Here's how the part is built. I have some questions about the finished solid (model axes, mm). Face numbers are marked on the shaded views. A direction names the side the tool comes from. Coordinates: 2 decimals unless noted, no trailing zeros. Write each loop counter-clockwise with the first axis right and the second up, starting at its lowest first coordinate (ties: lowest second). Pieces come first, ordered by that corner, then holes. Notation, with made-up numbers: M 14.5,-11 L 28.5,-11 A12 ccw 28.5,12 Z; hole C 19.5,33.25 d7. An arc over 180 degrees is marked long. Use a Markdown table: item, result.
```python
from build123d import *

# Parameters (mm, degrees)
CROQUIS1_W              = 111.196890842
CROQUIS1_H              = 104.63014532
SALIENTE_EXTRUIR1_DEPTH = 25
SALIENTE_EXTRUIR2_DEPTH = 25
MATRIZL4_COUNT          = 2
MATRIZL4_PITCH          = 50
MATRIZL5_COUNT          = 2
MATRIZL5_PITCH          = 50
CROQUIS3_R              = 50.793115706
CORTAR_EXTRUIR4_DEPTH   = 120


with BuildPart() as part:
    # Croquis1 → Saliente-Extruir1 (new body)
    with BuildSketch(Plane.XY):
        Rectangle(CROQUIS1_W, CROQUIS1_H)
    saliente_extruir1 = extrude(amount=SALIENTE_EXTRUIR1_DEPTH)

    # Croquis2 → Saliente-Extruir2 (add)
    with BuildSketch(Plane.XY.offset(25)):
        Polygon((-3.132824134, -80.10377536), (81.011557784, -3.059075666), (4.937773514, 80.024920806), (-79.206608404, 2.980221112), align=None)
    saliente_extruir2 = extrude(amount=SALIENTE_EXTRUIR2_DEPTH)

    # MatrizL4: Saliente-Extruir1, Saliente-Extruir2 ×2
    with Locations(*[(0, 0, i * MATRIZL4_PITCH) for i in range(1, MATRIZL4_COUNT)]):
        add(saliente_extruir1)
        add(saliente_extruir2)

    # MatrizL5: Saliente-Extruir2 ×2
    with Locations(*[(0, 0, -i * MATRIZL5_PITCH) for i in range(1, MATRIZL5_COUNT)]):
        add(saliente_extruir2)

    # Croquis3 → Cortar-Extruir4 (cut)
    with BuildSketch(Plane(origin=(0, 0, -25), x_dir=(-1, 0, 0), z_dir=(0, 0, -1))):
        Circle(CROQUIS3_R)
    extrude(amount=-CORTAR_EXTRUIR4_DEPTH, mode=Mode.SUBTRACT)


solid = part.part
```
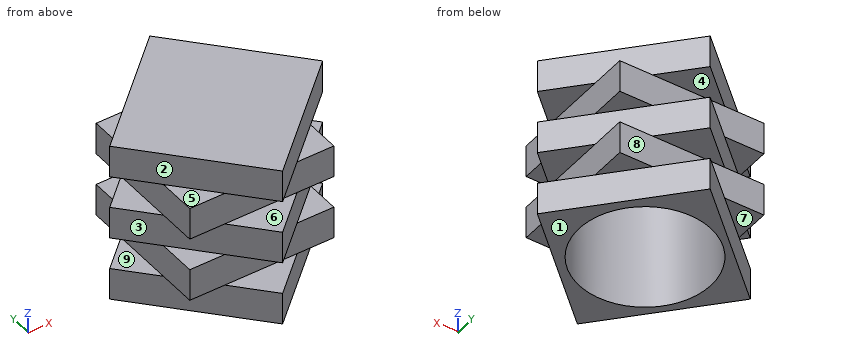
1. Suppose I cut it at C-C on x = -46. Write out the boundary of the cut face in (y, z), and give its area (3 significant figures).
Answers follow:
| item | result |
|---|---|
| outline | M -52.32,0 L -33.29,0 L -33.29,-25 L -21.54,-25 L -21.54,95 L 21.54,95 L 21.54,-25 L 33.39,-25 L 33.39,0 L 52.32,0 L 52.32,25 L 33.39,25 L 33.39,50 L 52.32,50 L 52.32,75 L 33.39,75 L 33.39,100 L -33.29,100 L -33.29,75 L -52.32,75 L -52.32,50 L -33.29,50 L -33.29,25 L -52.32,25 Z |
| area | 5,060 mm2 |
2. Suppose I cut it at B-B on z = 78. Write out the boundary of the cut face in (x, y).
Answers follow:
| item | result |
|---|---|
| outline | M -79.21,2.98 L -3.13,-80.1 L 81.01,-3.06 L 4.94,80.02 Z; hole C 0,0 d101.59 |
3. Suppose I cut it at A-A on y = -69.5. Write out the boundary of the cut face in (x, z).
Answers follow:
| item | result |
|---|---|
| outline | M -12.84,-25 L 8.45,-25 L 8.45,0 L -12.84,0 Z; M -12.84,25 L 8.45,25 L 8.45,50 L -12.84,50 Z; M -12.84,75 L 8.45,75 L 8.45,100 L -12.84,100 Z |
4. Will these pins go through, and if not, where does the flat tip stop? pin 1 Ø4 at (x, z) = (17, -5) entering from -Y; pin 2 Ø1 at (y, z) = (-11.5, 82) entering from +X; pin 3 Ø12 at (x, z) = (-2.5, 55) entering from +Y; pin 4 Ø6 at (y, z) = (62.5, 19.5) entering from -X.
Answers follow:
| item | result |
|---|---|
| pin 1 | stops at y = -63.5 |
| pin 2 | stops at x = 72.34 |
| pin 3 | stops at y = 76.25 |
| pin 4 | passes through |
5. Which directions (+Z, -Z, +X, -X, +Y, -Y) give clear straight access to the entire face, cutting with the end or side of a thin tool? Please do the marked faces 5, 6, 7, 8 and 9.
Answers follow:
| item | result |
|---|---|
| face 5 | +Z, -X, -Y |
| face 6 | +X, -X, -Y |
| face 7 | -Z, -X, +Y |
| face 8 | +X, -X, +Y |
| face 9 | -X, +Y, -Y |
6. I need wall thicknesses on probe 1 along Z at (x, y) = (67, -6); probe 2 along Y at (x, z) = (2, 22); probe 3 along Z at (x, y) = (-18, 26). Which ranges of each line are inside material? Lowest first, please.
Answers follow:
| item | result |
|---|---|
| probe 1 | z = -25 to 0, 25 to 50, 75 to 100 |
| probe 2 | y = -52.32 to -50.75, 50.75 to 52.32 |
| probe 3 | z = 95 to 100 |
7. We'd pull the mould along Z, two halves only. Please class the marked faces 1, 2, 3 and 4: +Z half, -Z half, draft (parallel to the pull), parting line (faces both ways), or undercut.
Answers follow:
| item | result |
|---|---|
| face 1 | -Z half |
| face 2 | draft |
| face 3 | undercut |
| face 4 | undercut |
8. Suppose I cut it at D-D on y = -18. Write out the boundary of the cut face in (x, z), and give its area (3 significant figures).
Answers follow:
| item | result |
|---|---|
| outline | M -60,-25 L -47.5,-25 L -47.5,95 L 47.5,95 L 47.5,-25 L 64.69,-25 L 64.69,0 L 55.6,0 L 55.6,25 L 64.69,25 L 64.69,50 L 55.6,50 L 55.6,75 L 64.69,75 L 64.69,100 L -60,100 L -60,75 L -55.6,75 L -55.6,50 L -60,50 L -60,25 L -55.6,25 L -55.6,0 L -60,0 Z |
| area | 3,510 mm2 |
